Source: three-view drawing plus pictorial views. Frame: mm from the lowest corner of the part. Give positions to 0.01 mm unless a question says otherwise; leave off trailing zeros. Write each loop counter-clockwise with the first axis right and the second up, starting at its lowest first coordinate (ties: lowest second). Pieces come first, ordered by that corner, then holes. Notation, with made-up numbers: M 67.5,43.25 L 95.5,43.25 A30 cw 95.5,70.25 Z; hole C 23,1 d11. An arc over 180 degrees is marked long. Return JSON: item names as keys, results as strings.
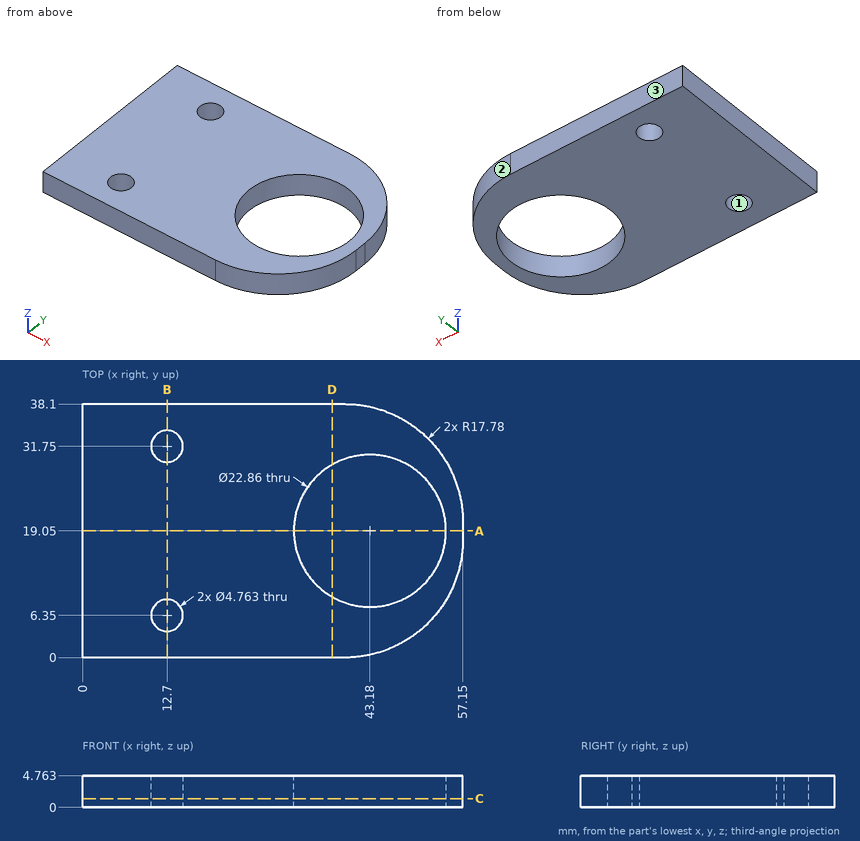
1) Line query: line 1 (X direction, y = 6, z = 1.55) (1 decimal); line 2 (X direction, y = 20, z = 0.95); line 3 (Y direction, x = 52.5, z = 1) (1 decimal). Output: solid intervals per line, ascending. Write a range as [from, to].
Numbers:
{"line 1": "x = [0, 10.3], [15.1, 52.7]", "line 2": "x = [0, 31.79], [54.57, 57.15]", "line 3": "y = [5.8, 12.4], [25.7, 32.3]"}
2) Cut plane B-B, the plane x = 12.7. Return the cut outline in (y, z), then the cut area to 3 significant figures.
Numbers:
{"outline": "M 0,0 L 3.97,0 L 3.97,4.76 L 0,4.76 Z; M 8.73,0 L 29.37,0 L 29.37,4.76 L 8.73,4.76 Z; M 34.13,0 L 38.1,0 L 38.1,4.76 L 34.13,4.76 Z", "area": "136 mm²"}
3) Cut plane D-D, the plane x = 37.5. Return the cut outline in (y, z).
Numbers:
{"outline": "M 0,0 L 9.13,0 L 9.13,4.76 L 0,4.76 Z; M 28.97,0 L 38.1,0 L 38.1,4.76 L 28.97,4.76 Z"}
4) Cut plane A-A, the plane y = 19.05. Return the cut outline in (x, z).
Numbers:
{"outline": "M 0,0 L 31.75,0 L 31.75,4.76 L 0,4.76 Z; M 54.61,0 L 57.15,0 L 57.15,4.76 L 54.61,4.76 Z"}
5) Cut plane C-C, the plane z = 1.3. Return the cut outline in (x, y).
Numbers:
{"outline": "M 0,0 L 39.37,0 A17.78 ccw 57.15,17.78 L 57.15,20.32 A17.78 ccw 39.37,38.1 L 0,38.1 Z; hole C 12.7,6.35 d4.76; hole C 12.7,31.75 d4.76; hole C 43.18,19.05 d22.86"}
6) Draft query along X for the marked faces 1, 2 and 3. Return one class per face: released by +X, released by -X, zero draft, split by the parting line, or undercut.
Numbers:
{"face 1": "undercut", "face 2": "released by +X", "face 3": "zero draft"}
